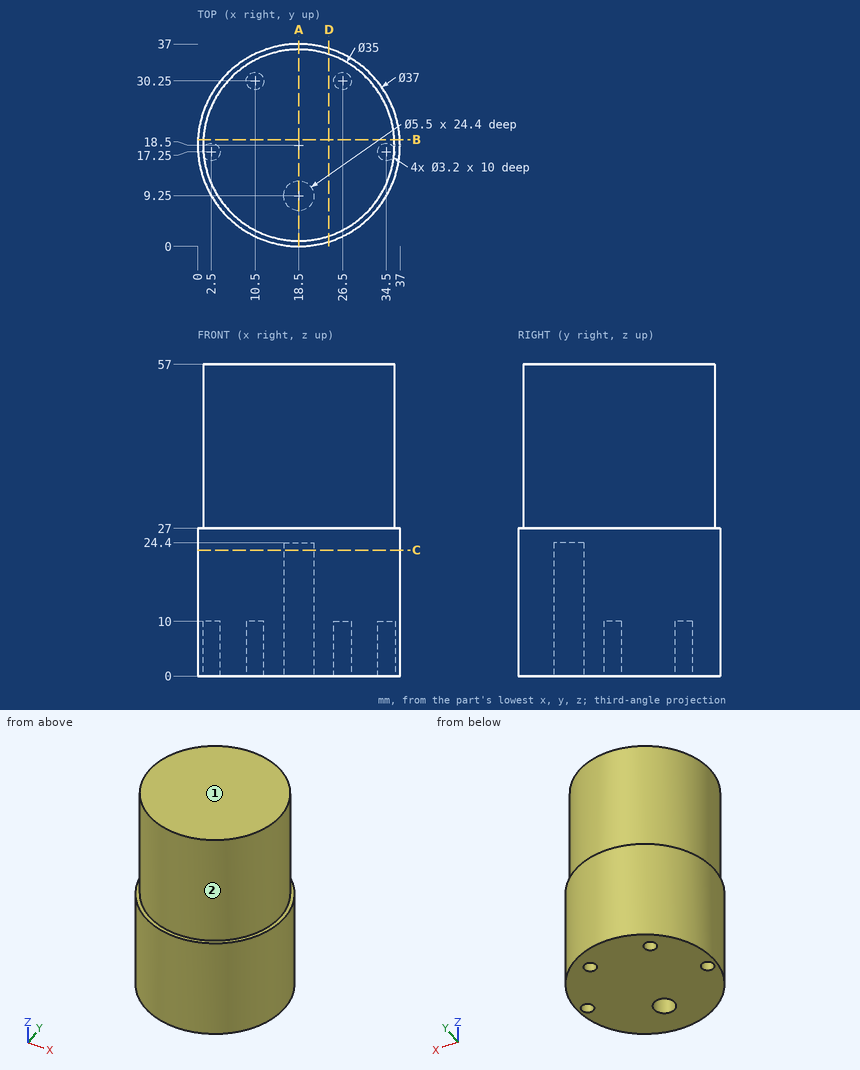
Print and shaded views of the part. All mm, measured from the part's lowest x, y and z. A direction names the side the tool comes from. Give positions to 0.01 mm unless a question says otherwise; leave off trailing zeros. Write each loop counter-clockwise with the first axis right and the second up, starting at its lowest first coordinate (ties: lowest second). Pieces come first, ordered by that corner, then holes. Notation, with made-up numbers: (2, 9.5) -> (40, 9.5) arc R19 cw to (40, 19.5) -> close; hole circle Ø10 at (33, 88). An arc over 180 degrees is marked (long way). Use CSV: the item, a comma, the result in double quotes. Start each with the question number.
1) Drill centre lines: L1, parallel to X at y = 30, z = 7; L2, parallel to X at y = 17, z = 7.5; L3, parallel to Z at x = 31, y = 6. Where is each one in solid material? Low to high.
2) Cut at A-A on x = 18.5. List the corners of the cut face in (y, z), plus the area to 3 significant figures.
3) Pin check, flat tips, straight feed: P1, Ø1, axis at x = 3, y = 17.5, coming from the -Z side; P2, Ø12, axis at y = 28, z = 30, coming from the +X side; P3, Ø2, axis at x = 6.5, z = 29.5, coming from the -Y side. Stop position of each tip, or through.
4) Cut at D-D on x = 24. List the corners of the cut face in (y, z).
5) Cut at C-C on z = 23. List the corners of the cut face in (x, y), plus the area to 3 significant figures.
6) Cut at B-B on y = 19.5. List the corners of the cut face in (x, z), plus the area to 3 significant figures.
7) Tool access for the marked faces 1 and 2: list every direction of +Z, -Z, +X, -X, +Y, -Y with a clear straight run to the whole face (end or side of a thin tool).
Final values:
1,L1,"x = 4.01 to 8.92, 12.08 to 24.92, 28.08 to 32.99"
1,L2,"x = 0.06 to 0.92, 4.08 to 32.92, 36.08 to 36.94"
1,L3,"z = 0 to 27"
2,outline,"(0, 0) -> (6.5, 0) -> (6.5, 24.4) -> (12, 24.4) -> (12, 0) -> (37, 0) -> (37, 27) -> (36, 27) -> (36, 57) -> (1, 57) -> (1, 27) -> (0, 27) -> close"
2,area,"1,910 mm2"
3,P1,"stops at z = 10"
3,P2,"stops at x = 36.49"
3,P3,"stops at y = 4.89"
4,outline,"(0.84, 0) -> (36.16, 0) -> (36.16, 27) -> (35.11, 27) -> (35.11, 57) -> (1.89, 57) -> (1.89, 27) -> (0.84, 27) -> close"
5,outline,"circle Ø37 at (18.5, 18.5); hole circle Ø5.5 at (18.5, 9.25)"
5,area,"1,050 mm2"
6,outline,"(0.03, 0) -> (36.97, 0) -> (36.97, 27) -> (35.97, 27) -> (35.97, 57) -> (1.03, 57) -> (1.03, 27) -> (0.03, 27) -> close"
6,area,"2,050 mm2"
7,face 1,"+Z, +X, -X, +Y, -Y"
7,face 2,"+Z"
